Design review of the part built by this model. Coordinates are the model's own, in mm. Coordinates: 2 decimals unless noted, no trailing zeros. Loops run counter-clockwise (first coordinate to the right, second up) from the corner with the lowest first, then second, coordinate; pieces in that order, holes last. Notation, with made-up numbers: (80, 29.5) -> (133, 29.5) arc R32 ccw to (133, 59.5) -> close; hole circle Ø1 at (55, -6.75). An arc over 180 degrees is marked (long way). Answer in a Markdown table with one row per item.
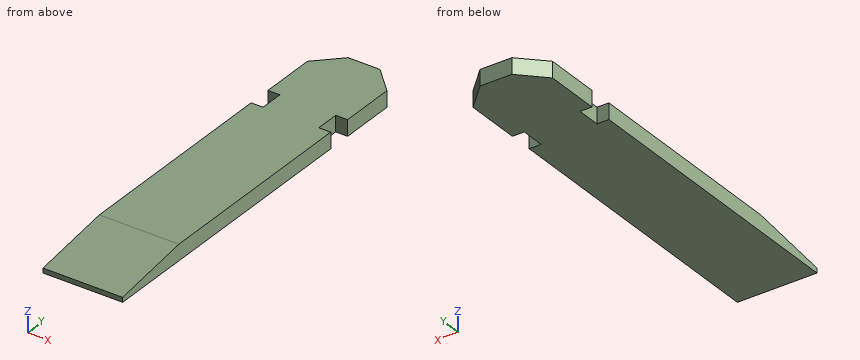
```python
from build123d import *

# Parameters (mm, degrees)
SKETCH_W        = 10
SKETCH_H        = 50
PAD_DEPTH       = 2
SKETCH001_W     = 1.5
SKETCH001_H     = 3
POCKET_DEPTH    = 3
CHAMFER_ANGLE   = 8
CHAMFER_SIZE    = 10
CHAMFER001_SIZE = 3


with BuildPart() as part:
    # Sketch → Pad (new body)
    with BuildSketch(Plane.XY):
        with Locations((5, 25)):
            Rectangle(SKETCH_W, SKETCH_H)
    extrude(amount=PAD_DEPTH)

    # Sketch001 (on Face6 of Pad) → Pocket (cut)
    with BuildSketch(Plane.XY.offset(2)):
        with Locations((9.25, 38.5)):
            Rectangle(SKETCH001_W, SKETCH001_H)
        with Locations((0.75, 38.5)):
            Rectangle(SKETCH001_W, SKETCH001_H)
    extrude(amount=-POCKET_DEPTH, mode=Mode.SUBTRACT)

    # Chamfer
    chamfer_edges = [part.edges().sort_by_distance(p)[0] for p in [
        (5, 0, 2),
    ]]
    chamfer_side = part.faces().sort_by_distance((5, 24.752546, 2))[0]
    chamfer(chamfer_edges, length=CHAMFER_SIZE, angle=CHAMFER_ANGLE, reference=chamfer_side)

    # Chamfer001
    chamfer001_edges = [part.edges().sort_by_distance(p)[0] for p in [
        (0, 50, 1),
        (10, 50, 1),
    ]]
    chamfer(chamfer001_edges, length=CHAMFER001_SIZE)


solid = part.part
```
(1) To check wall thickness, follow probe 1 along Z at (x, y) = (0.5, 5); probe 2 along Y at (x, z) = (2.75, 0.5); probe 3 along Z at (x, y) = (5.75, 3). State the ranges of each line that lie inside material, in increasing order.
Evaluation:
| item | result |
|---|---|
| probe 1 | z = 0 to 1.3 |
| probe 2 | y = 0 to 49.75 |
| probe 3 | z = 0 to 1.02 |
(2) Take a section at A-A on x = 2.25. Give the boundary of the cut face in (y, z), and give its area (3 significant figures).
Evaluation:
| item | result |
|---|---|
| outline | (0, 0) -> (49.25, 0) -> (49.25, 2) -> (10, 2) -> (0, 0.59) -> close |
| area | 91.5 mm² |
(3) For pin 1 (0.6 mm diameter, centred on y = 38, z = 0.5, fed in from -X); pin 2 (1.2 mm diameter, centred on x = 9, z = 1.5, fed in from +Y); pin 3 (0.6 mm diameter, centred on y = 38.5, z = 1, fed in from +X), all flat-tipped, find the tip position at first contact; note any pin that passes through.
Evaluation:
| item | result |
|---|---|
| pin 1 | stops at x = 1.5 |
| pin 2 | stops at y = 48.6 |
| pin 3 | stops at x = 8.5 |
(4) Take a section at B-B on z = 1. Give the boundary of the cut face in (x, y).
Evaluation:
| item | result |
|---|---|
| outline | (0, 2.88) -> (10, 2.88) -> (10, 37) -> (8.5, 37) -> (8.5, 40) -> (10, 40) -> (10, 47) -> (7, 50) -> (3, 50) -> (0, 47) -> (0, 40) -> (1.5, 40) -> (1.5, 37) -> (0, 37) -> close |
(5) Take a section at C-C on y = 9. Give the boundary of the cut face in (x, z).
Evaluation:
| item | result |
|---|---|
| outline | (0, 0) -> (10, 0) -> (10, 1.86) -> (0, 1.86) -> close |
(6) Take a section at D-D on x = 8. Give the boundary of the cut face in (y, z).
Evaluation:
| item | result |
|---|---|
| outline | (0, 0) -> (49, 0) -> (49, 2) -> (10, 2) -> (0, 0.59) -> close |
